Work out the finished part from the listing and answer in its coordinate system (mm). A direction names the side the tool comes from. Round coordinates to 2 decimals unless told otherwise and drop trailing zeros. Order: outer loops, then holes, each group sorted by start corner. A loop starts at its lowest first (then second) coordinate and runs counter-clockwise, first axis right, second up.
Autodesk Inventor part; units mm, degrees
ref_plane "YZ Plane" through (0, 0, 0) normal (1, 0, 0) x (0, 1, 0)
ref_plane "XZ Plane" through (0, 0, 0) normal (0, 1, 0) x (-1, 0, 0)
ref_plane "XY Plane" through (0, 0, 0) normal (0, 0, 1) x (1, 0, 0)
sketch "Boceto1" plane through (0, 0, 0) normal (0, 1, 0) x (-1, 0, 0)
  circle A0 centre (0, 0) radius 46.5
  dimension "d0" = 93
extrude "Extrusión1" add sketch "Boceto1" along normal blind 45
sketch "Boceto2" plane through (0, 0, 0) normal (0, -1, 0) x (1, 0, 0)
  point P0 (0, 0)
sketch "Boceto3" plane through (0, 45, 0) normal (0, 1, 0) x (1, 0, 0)
  line L0 (46.5, -15) -> (-46.6883, -15)
  circle A0 centre (0, 0) radius 46.5
  line L1 (46.5, -15) -> (46.5, 15)
  line L2 (46.5, 0) -> (46.5, -15)
  line L3 (46.5, 0) -> (46.5, 15)
  line L4 (-46.6883, -15) -> (-46.6883, 15)
  line L5 (-46.6883, 15) -> (46.5, 15)
extrude "Extrusión2" cut sketch "Boceto3" against normal blind 30 contours L0 A0 L1 | L0 A0 L5 | A0 L5 L1 | L0 L4 L5 A0
sketch "Boceto4" plane through (0, 45, 0) normal (0, 1, 0) x (1, 0, 0)
  circle A0 centre (0, 0) radius 46.5
  point P0 (-44.0142, -15)
  point P1 (44.0142, -15)
sketch "Boceto5" plane through (0, 45, 0) normal (0, 1, 0) x (1, 0, 0)
  line L0 (-20.0239, -77.8543) -> (-20, -77.821)
  point P0 (0, 0)
  point P1 (-20, -41.9792)
  point P2 (0, 0)
  point P3 (0, 0)
extrude "Extrusión3" [suppressed]
sketch "Boceto6" plane through (0, 45, 0) normal (0, 1, 0) x (1, 0, 0)
  point P0 (0, 0)
sketch "Boceto7" plane through (0, 45, 0) normal (0, 1, 0) x (1, 0, 0)
  point P0 (0, 0)
sketch "Boceto8" plane through (0, 45, 0) normal (0, 1, 0) x (1, 0, 0)
  point P0 (0, 0)
sketch "Boceto9" plane through (0, 0, 0) normal (0, -1, 0) x (1, 0, 0)
  arc A0 (-44.0142, -15) -> (-44.0142, 15) centre (0, 0) ccw
  point P0 (5, 46.2304)
  point P1 (19.0142, 42.4348)
hole "Agujero1" at (0, 0, 0) direction (0, 1, 0) diameter 3.5 depth 10
sketch "Boceto10" plane through (0, 0, 0) normal (0, -1, 0) x (1, 0, 0)
  point P0 (0, 0)
sketch "Boceto11" plane through (0, 0, 0) normal (0, -1, 0) x (1, 0, 0)
  point P0 (0, 0)
sketch "Boceto12" plane through (0, 0, 0) normal (0, -1, 0) x (1, 0, 0)
  line L0 (1.5, -0.9014) -> (-1.5, -0.9014)
  arc A0 (-1.5, -0.9014) -> (1.5, -0.9014) centre (0, 0) ccw
extrude "Extrusión4" add sketch "Boceto12" against normal blind 10
sketch "Boceto13" plane through (5, 40, 88) normal (0, 0, 1) x (1, 0, 0)
  point P0 (-5, -40)
  point P1 (39.0142, 0)
sketch "Boceto14" plane through (5, 40, 88) normal (0, 0, 1) x (1, 0, 0)
  point P0 (-5, -40)
sketch "Boceto15" plane through (5, 40, 88) normal (0, 0, 1) x (1, 0, 0)
  point P0 (-5, -40)
  point P1 (39.0142, 0)
sketch "Boceto16" plane through (5, 40, 88) normal (0, 0, 1) x (1, 0, 0)
  point P0 (-5, -40)
  point P1 (0, 0)
  point P2 (39.0142, 0)
sketch "Boceto17" plane through (5, 40, 88) normal (0, 0, 1) x (1, 0, 0)
  point P0 (-5, -40)
  point P1 (39.0586, 0)
  point P2 (0, 0)
sketch "Boceto18" plane through (5, 40, 88) normal (0, 0, 1) x (1, 0, 0)
  line L0 (0, -40) -> (0, 0)
  line L1 (39.0142, -40) -> (0, -40)
  line L2 (39.0142, 20) -> (39.0142, -40)
  line L3 (0, 20) -> (0, -40)
  line L4 (0, -40) -> (39.0142, -40)
  line L5 (0, 20) -> (2, 20)
  line L6 (39.0142, 20) -> (38, 20)
  arc A0 (2, 20) -> (38, 20) centre (20, 18.1) ccw
  point P0 (-5, -40)
extrude "Extrusión5" [suppressed]
sketch "Boceto19" plane through (0, 15, 0) normal (0, 1, 0) x (1, 0, 0)
  point P0 (0, 0)
sketch "Boceto20" plane through (0, 45, 0) normal (0, 1, 0) x (1, 0, 0)
  point P0 (0, 0)
sketch "Boceto21" plane through (0, 45, 0) normal (0, 1, 0) x (1, 0, 0)
  point P0 (0, 0)
sketch "Boceto22" plane through (0, 45, 0) normal (0, 1, 0) x (1, 0, 0)
  point P0 (0, 0)
sketch "Boceto23" plane through (19.0142, 40, 67.4096) normal (0, 0, 1) x (1, 0, 0)
  line L0 (25, 0) -> (-63.0284, 0)
  point P0 (-19.0142, -40)
sketch "Boceto24" plane through (0, 45, 0) normal (0, 1, 0) x (1, 0, 0)
  arc A0 (-1.5, 0.9014) -> (1.5, 0.9014) centre (0, 0) ccw
  arc A1 (15.0142, -44.0094) -> (44.0142, -15) centre (0, 0) ccw
  circle A2 centre (0, 0) radius 46.5
  arc A3 (-44.0142, -15) -> (44.0142, -15) centre (0, 0) ccw
  line L0 (44.0142, -15) -> (44.0142, -67.5)
  line L1 (44.0142, -67.5) -> (15.0142, -67.5)
  line L2 (15.0142, -67.5) -> (15.0142, -44.0094)
extrude "Extrusión6" add sketch "Boceto24" against normal blind 40 contours A1 L0 L1 L2
sketch "Boceto25" plane through (15.0142, 45, 67.5) normal (0, 0, 1) x (1, 0, 0)
  line L0 (29, 0) -> (29, 12.5)
  line L1 (29, 12.5) -> (27, 12.5)
  line L2 (0, 12.5) -> (2, 12.5)
  arc A0 (2, 12.5) -> (27, 12.5) centre (14.5, 12.5) ccw
  line L3 (29, -40) -> (0, -40)
  line L4 (0, 12.5) -> (0, -40)
  line L5 (0, -40) -> (29, -40)
  line L6 (29, -40) -> (29, 0)
  point P0 (0, 0)
sketch "Boceto26" plane through (0, 45, 0) normal (0, 1, 0) x (1, 0, 0)
  point P0 (0, 0)
extrude "Extrusión7" add sketch "Boceto25" against normal blind 52.5
sketch "Boceto27" plane through (15.0142, 5, 67.5) normal (0, 0, 1) x (1, 0, 0)
  point P0 (-15.0142, -5)
sketch "Boceto28" plane through (15.0142, 5, 67.5) normal (0, 0, 1) x (1, 0, 0)
  line L0 (0, 0) -> (0, -5)
  line L1 (29, 0) -> (29, -5)
  line L2 (29, -5) -> (0, -5)
  line L3 (0, 0) -> (29, 0)
  line L4 (29, 0) -> (0, 0)
  point P0 (-15.0142, -5)
extrude "Extrusión8" add sketch "Boceto28" against normal blind 70
properties part number "cilindro"
Item 1: A tool of negligible diameter and unlimited length cuts with its end or side. For faces 5 (the face through (-8, 45, 27)), 6 (the face through (-0.05, 5.07, 1.75)), 7 (the face through (-1, 30, -15)), from which of +Z, -Z, +X, -X, +Y, -Y can it reach the whole face along a straight path? Write none if from no direction.
Item 2: For a pull along Z with two mould halves and no side action, classify faces 1 (the face through (0, 5, -0.901)), 2 (the face through (15.014, 36, 53)), 3 (the face through (1, 32, 15)), 4 (the face through (29, 23, 67.5)) as released by +Z, released by -Z, zero draft, split by the parting line, or undercut.
Item 3: Find the intervals of material crossed by line 1 along X through (y, z) = (4.75, 0); line 2 along Z through (x, y) = (0, 3.75); line 3 along Y through (x, z) = (-27.5, 19.5), in increasing order.
Item 4: Find section A-A (x = 0). Write down the section's boundary in (y, z), plus the area to 3 significant figures.
Item 5: Find section D-D (x = -22.5). Write down the section's boundary in (y, z), plus the area to 3 significant figures.
Item 6: Given pin 1 (1 mm diameter, centred on x = 30, z = -6, fed in from +Y); pin 2 (4 mm diameter, centred on x = -2, z = 16.5, fed in from +Y); pin 3 (4 mm diameter, centred on x = 24, y = 25, fed in from -Z), each flat-ended and moving along its own axis, determine where each tip first touches the part or whether it passes through.
Item 7: Find section C-C (z = 34). Write down the section's boundary in (x, y), plus the area to 3 significant figures.
Item 8: Find section B-B (y = 20.5). Write down the section's boundary in (x, z), plus the area to 3 significant figures.
Model answer:
1. face 5: +Z, -Z, -X, +Y
1. face 6: -Y
1. face 7: +X, -X, +Y
2. face 1: undercut
2. face 2: zero draft
2. face 3: undercut
2. face 4: released by +Z
3. line 1: x = -46.5 to -1.75, 1.75 to 46.5
3. line 2: z = -46.5 to -0.9, 1.75 to 46.5
3. line 3: y = 0 to 45
4. outline: (0, -46.5) - (45, -46.5) - (45, -15) - (15, -15) - (15, 15) - (45, 15) - (45, 46.5) - (0, 46.5) - (0, 1.75) - (10, 1.75) - (10, -0.9) - (0, -0.9) - close
4. area: 3,260 mm2
5. outline: (0, -40.69) - (45, -40.69) - (45, -15) - (15, -15) - (15, 15) - (45, 15) - (45, 40.69) - (0, 40.69) - close
5. area: 2,760 mm2
6. pin 1: stops at y = 15
6. pin 2: stops at y = 45
6. pin 3: stops at z = -40.97
7. outline: (-31.72, 0) - (44.01, 0) - (44.01, 57.5) - (42.01, 57.5) arc R12.5 cw to (17.01, 57.5) - (15.01, 57.5) - (15.01, 45) - (-31.72, 45) - close
7. area: 3,530 mm2
8. outline: (-44.01, -15) arc R46.5 ccw to (44.01, -15) - close; (-44.01, 15) - (44.01, 15) - (44.01, 67.5) - (15.01, 67.5) - (15.01, 44.01) arc R46.5 ccw to start
8. area: 5,020 mm2
